from build123d import *

# Parameters (mm, degrees)
EXTRUDE_1_DEPTH                 = 7.5
EXTRUDE_1_DEPTH_BACK            = 7.5
SKETCH_1_R                      = 3.5
CUT_EXTRUDE_1_REACH             = 10.986
SKETCH_2_W                      = 2.5
SKETCH_2_H                      = 4
CUT_EXTRUDE_1_DIRECTION_2_REACH = 10.986
FILLET_1_R                      = 0.2


with BuildPart() as part:
    # 草图1 → 凸台-拉伸1 (new, two sides: drawn at the far end of the back side and taken through both)
    with BuildSketch(Plane.XY.offset(-EXTRUDE_1_DEPTH_BACK)):
        Circle(SKETCH_1_R)
        with BuildLine():
            Line((-1.25, 1.5612495), (-1.25, -1.5612495))
            ThreePointArc((-1.25, -1.5612495), (0, -2), (1.25, -1.5612495))
            Line((1.25, -1.5612495), (1.25, 1.5612495))
            ThreePointArc((1.25, 1.5612495), (0, 2), (-1.25, 1.5612495))
        make_face(mode=Mode.SUBTRACT)
    extrude(amount=EXTRUDE_1_DEPTH + EXTRUDE_1_DEPTH_BACK)

    # 草图2 → 切除-拉伸1 (cut, up to next)
    with BuildSketch(Plane(origin=(0, 0, 0), x_dir=(1, 0, 0), z_dir=(0, 1, 0)), mode=Mode.PRIVATE) as cut_extrude_1_sk1:
        Rectangle(SKETCH_2_W, SKETCH_2_H)
    cut_extrude_1_tool1 = extrude(cut_extrude_1_sk1.sketch, amount=-CUT_EXTRUDE_1_REACH, mode=Mode.PRIVATE) & part.part
    add(cut_extrude_1_tool1.solids().sort_by_distance((0, 0, 0))[0], mode=Mode.SUBTRACT)

    # 草图2 → 切除-拉伸1 direction 2 (cut, up to next)
    with BuildSketch(Plane(origin=(0, 0, 0), x_dir=(1, 0, 0), z_dir=(0, 1, 0)), mode=Mode.PRIVATE) as cut_extrude_1_direction_2_sk1:
        Rectangle(SKETCH_2_W, SKETCH_2_H)
    cut_extrude_1_direction_2_tool1 = extrude(cut_extrude_1_direction_2_sk1.sketch, amount=CUT_EXTRUDE_1_DIRECTION_2_REACH, mode=Mode.PRIVATE) & part.part
    add(cut_extrude_1_direction_2_tool1.solids().sort_by_distance((0, 0, 0))[0], mode=Mode.SUBTRACT)

    # 圆角1
    fillet_1_edges = [part.edges().sort_by_distance(p)[0] for p in [
        (-3.5, 0, -7.5),
        (-3.5, 0, 7.5),
    ]]
    fillet(fillet_1_edges, radius=FILLET_1_R)


solid = part.part
Part model, mm, in its own coordinate system. A direction names the side the tool comes from. Coordinates: 2 decimals unless noted, no trailing zeros. Loops run counter-clockwise (first coordinate to the right, second up) from the corner with the lowest first, then second, coordinate; pieces in that order, holes last. Notation, with made-up numbers: (33.5, -30.75) -> (86.5, -30.75) arc R10 ccw to (86.5, -11.75) -> close; hole circle Ø9 at (-21.5, -14.75). An arc over 180 degrees is marked (long way). Use a Markdown table: item, result. Add a question column.
Item 1: Band-saw the part on B-B on y = 0. Write the cut outline in (x, z), plus the area to 3 significant figures.
Item 2: Band-saw the part on C-C on z = -5.75. Write the cut outline in (x, y), plus the area to 3 significant figures.
Item 3: Flat gauge pins, fed straight in: P1, Ø4, axis at x = 2, z = 1, coming from the +Y side; P2, Ø1.5, axis at x = -2.5, z = -4.5, coming from the -Y side; P3, Ø2, axis at y = 0.5, z = 1.5, coming from the +X side. Where does each tip first touch, or does it go through?
Item 4: Which spindle directions (+Z, -Z, +X, -X, +Y, -Y) get a long thin tool onto all of the face, cutting with end or side? Do faces 4 (the flat face through (0, 3, -2)), 5 (the cylindrical face through (0, -2, -5)), 6 (the flat face through (1.25, 0, 0)), 7 (the flat face through (1.42, 0.05, -7.5)), 8 (the flat face through (1.42, 0.05, 7.5)). Say none if no direction does.
Item 5: Pull direction Y, two halves, no side cores. Call faces 1 (the flat face through (0, 3, 2)), 2 (the cylindrical face through (0, 2, -5)), 3 (the cylindrical face through (3.233, -1.341, -0.102)): +Y half, -Y half, draft (parallel to the pull), parting line (faces both ways), or undercut.
Item 6: Band-saw the part on A-A on x = 0. Write the cut outline in (y, z), plus the area to 3 significant figures.
Item 7: Probe probe 1 along X at (y, z) = (-1.25, 4.25); probe 2 along Z at (x, y) = (0.75, 3); probe 3 along X at (y, z) = (1.75, 1). List the from-to ranges inside material, lowest first.
Geometry says:
| question | item | result |
|---|---|---|
| 1 | outline | (-3.5, -7.3) arc R0.2 ccw to (-3.3, -7.5) -> (-1.25, -7.5) -> (-1.25, 7.5) -> (-3.3, 7.5) arc R0.2 ccw to (-3.5, 7.3) -> close; (1.25, -7.5) -> (3.3, -7.5) arc R0.2 ccw to (3.5, -7.3) -> (3.5, 7.3) arc R0.2 ccw to (3.3, 7.5) -> (1.25, 7.5) -> close |
| 1 | area | 67.5 mm² |
| 2 | outline | circle Ø7 at (0, 0); hole (-1.25, -1.56) arc R2 ccw to (1.25, -1.56) -> (1.25, 1.56) arc R2 ccw to (-1.25, 1.56) -> close |
| 2 | area | 29.2 mm² |
| 3 | P1 | y = 3.49 |
| 3 | P2 | y = -3.03 |
| 3 | P3 | x = 3.5 |
| 4 | face 4 | +Y, -Y |
| 4 | face 5 | +Z, -Z |
| 4 | face 6 | none |
| 4 | face 7 | -Z, +X, -X, +Y, -Y |
| 4 | face 8 | +Z, +X, -X, +Y, -Y |
| 5 | face 1 | draft |
| 5 | face 2 | undercut |
| 5 | face 3 | parting line |
| 6 | outline | (-3.5, -7.3) arc R0.2 ccw to (-3.3, -7.5) -> (-2, -7.5) -> (-2, -2) -> (-3.5, -2) -> close; (-3.5, 2) -> (-2, 2) -> (-2, 7.5) -> (-3.3, 7.5) arc R0.2 ccw to (-3.5, 7.3) -> close; (2, -7.5) -> (3.3, -7.5) arc R0.2 ccw to (3.5, -7.3) -> (3.5, -2) -> (2, -2) -> close; (2, 2) -> (3.5, 2) -> (3.5, 7.3) arc R0.2 ccw to (3.3, 7.5) -> (2, 7.5) -> close |
| 6 | area | 33.0 mm² |
| 7 | probe 1 | -3.27 to -1.25, 1.25 to 3.27 |
| 7 | probe 2 | -7.5 to -2, 2 to 7.5 |
| 7 | probe 3 | -3.03 to -1.25, 1.25 to 3.03 |
